Model file for the job. Use its own axes, mm. A direction names the side the tool comes from. Coordinates: 2 decimals unless noted, no trailing zeros. Order: outer loops, then holes, each group sorted by start corner. A loop starts at its lowest first (then second) coordinate and runs counter-clockwise, first axis right, second up. Notation, with made-up numbers: (-33, 42) -> (-3, 42) arc R20 cw to (-3, 65) -> close; hole circle Ø10 at (77.25, 50). An arc over 180 degrees is marked (long way). Write item = value, one per line. Start each with the question number.
Q1. Cut at B-B, the plane z = 0.9. List the corners of the cut face in (x, y), plus the area to 3 significant figures.
Q2. 3-axis set-ups, long thin cutter, end or side, ignore diameter. For faces 5 (the face through (7.259, 4.454, 2.465)), 6 (the face through (12.83, 2.1, 2.47)), 7 (the face through (48, 4.906, 4)), 8 (the face through (17.904, 8.634, 3.745)), 9 (the face through (47, 9.406, 2)): which of +Z, -Z, +X, -X, +Y, -Y reach the whole face in a straight line?
Q3. Cut at D-D, the plane x = 74.5. List the corners of the cut face in (y, z).
Q4. Cut at A-A, the plane x = 27.5. List the corners of the cut face in (y, z), plus the area to 3 significant figures.
Q5. Flat gauge pins, fed straight in: pin 1 (0.8 mm diameter, centred on x = 45.5, y = 9, fed in from +Z); pin 2 (0.7 mm diameter, centred on x = 46, z = 3.5, fed in from +Y); pin 3 (0.7 mm diameter, centred on x = 44.5, z = 4, fed in from -Y). Where does each tip first touch, or does it go through?
Q6. Wall check: line 1 (X direction, y = 6.25, z = 3.1); line 2 (Y direction, x = 41, z = 1.9); line 3 (X direction, y = 5, z = 2.95). Give the ranges that are in metal, low to high. Write a range as from..to.
Q7. Cut at C-C, the plane x = 8. List the corners of the cut face in (y, z), plus the area to 3 significant figures.
Q8. Mould opens along Y. For faces 1 (the face through (0.83, 6.24, 2.46)), 2 (the face through (46, 6, 0)), 3 (the face through (48, 7.906, 4)), 4 (the face through (88.824, 6.494, 2.465)) say: +Y half, -Y half, draft (parallel to the pull), parting line (faces both ways), or undercut.
Solid Edge part; units mm, degrees
sketch "Sketch1" plane through (0, 0, 0) normal (0, 0, -1) x (-1, 0, 0)
  circle A0 centre (-6.8258, 6.406) radius 2
  line L0 (-76.7103, 9.406) -> (-16.7103, 9.406)
  line L1 (-16.7103, 9.406) -> (-8.8158, 12.0664)
  line L2 (-16.7103, 3.406) -> (-8.8333, 0.7518)
  line L3 (-16.7103, 3.406) -> (-76.7103, 3.406)
  line L4 (-76.7103, 3.406) -> (-84.3711, 0.9311)
  line L5 (-85.2395, 12.1925) -> (-76.7103, 9.406)
  arc A1 (-8.8158, 12.0664) -> (-8.8333, 0.7518) centre (-6.8258, 6.406) cw
  arc A2 (-84.3711, 0.9311) -> (-85.2395, 12.1925) centre (-86.8258, 6.406) cw
  circle A3 centre (-86.8258, 6.406) radius 2
  dimension "D1" = 76.7103
  dimension "D2" = 16.7103
extrude "Protrusion1" add sketch "Sketch1" against normal blind 5
sketch "Sketch2" plane through (46.7103, 3.406, 2.5) normal (0, -1, 0) x (1, 0, 0)
  line L0 (-34.5366, 2.906) -> (-24.5967, 0.0249)
  line L1 (-24.5967, 0.0249) -> (24.6704, 0.0249)
  line L2 (24.6704, 0.0249) -> (35.7626, 2.906)
extrude "Enlèvement_matière_1" cut sketch "Sketch2" against normal blind 1.5 and the other way through all material side at (17.1576, 3.406, 4.0135)
sketch "Sketch3" plane through (46.7103, 9.406, 2.5) normal (0, 1, 0) x (-1, 0, 0)
  line L0 (-24.6704, 0.0249) -> (-34.1994, 2.5)
  line L1 (24.5967, 0.0249) -> (-24.6704, 0.0249)
  line L2 (33.1357, 2.5) -> (24.5967, 0.0249)
extrude "Enlèvement_matière_2" cut sketch "Sketch3" against normal blind 1.5 and the other way blind 16.364 material side at (76.1326, 9.406, 3.8108)
properties part number "AC_1.05"
Here are the results:
q1.outline = (8.82, 12.07) arc R6 ccw (long way) to (8.83, 0.75) -> (16.71, 3.41) -> (76.71, 3.41) -> (84.37, 0.93) arc R6 ccw (long way) to (85.24, 12.19) -> (76.71, 9.41) -> (16.71, 9.41) -> close; hole circle Ø4 at (6.83, 6.41); hole circle Ø4 at (86.83, 6.41)
q1.area = 633 mm²
q2.face_5 = +Z, -Z
q2.face_6 = +Z, -Z, -Y
q2.face_7 = +Z, -Y
q2.face_8 = +Z, +Y
q2.face_9 = +Z, -Z, +Y
q3.outline = (3.41, 0) -> (9.41, 0) -> (9.41, 3.34) -> (7.91, 3.34) -> (7.91, 5) -> (4.91, 5) -> (4.91, 3.34) -> (3.41, 3.34) -> close
q4.outline = (3.41, 0) -> (9.41, 0) -> (9.41, 2.52) -> (7.91, 2.52) -> (7.91, 5) -> (4.91, 5) -> (4.91, 2.52) -> (3.41, 2.52) -> close
q4.area = 22.6 mm²
q5.pin_1 = 2.52
q5.pin_2 = 7.91
q5.pin_3 = 4.91
q6.line_1 = 0.83..4.83, 8.82..84.83, 88.82..92.82
q6.line_2 = 3.41..9.41
q6.line_3 = 0.99..5.4, 8.25..85.4, 88.25..92.66
q7.outline = (0.52, 0) -> (4.79, 0) -> (4.79, 5) -> (0.52, 5) -> close; (8.03, 0) -> (12.29, 0) -> (12.29, 5) -> (8.03, 5) -> close
q7.area = 42.6 mm²
q8.face_1 = parting line
q8.face_2 = draft
q8.face_3 = +Y half
q8.face_4 = undercut
